CAD build for the part. Positions are in the model's coordinates, mm. A direction names the side the tool comes from. Give positions to 0.01 mm unless a question says otherwise; leave off trailing zeros. Write each loop counter-clockwise with the first axis right and the second up, starting at its lowest first coordinate (ties: lowest second). Pieces come first, ordered by that corner, then holes. Notation, with made-up numbers: (-15.75, -32.5) - (40.25, -32.5) arc R24 ccw to (40.25, -5.5) - close; hole circle Ø6 at (86, 69). An arc over 180 degrees is marked (long way). Answer as a JSON object with one key per item and string values.
Autodesk Inventor part; units mm, degrees
ref_plane "YZ Plane" through (0, 0, 0) normal (1, 0, 0) x (0, 1, 0)
ref_plane "XZ Plane" through (0, 0, 0) normal (0, 1, 0) x (-1, 0, 0)
ref_plane "XY Plane" through (0, 0, 0) normal (0, 0, 1) x (1, 0, 0)
sketch "Sketch1" plane through (0, 0, 0) normal (0, 0, 1) x (1, 0, 0)
  line L0 (-90, -12.5) -> (90, -12.5)
  line L1 (90, -12.5) -> (90, 12.5)
  line L2 (90, 12.5) -> (-90, 12.5)
  line L3 (-90, 12.5) -> (-90, -12.5)
  point P0 (0, 0)
  dimension "d0" = 25
  dimension "d1" = 12.5
  dimension "d2" = 180
  dimension "d3" = 90
extrude "Extrusion1" add sketch "Sketch1" along normal blind 1.6
fillet "Fillet1" radius 3 4 edges at (-90, -12.5, 0.8) (-90, 12.5, 0.8) (90, -12.5, 0.8) (90, 12.5, 0.8)
sketch "Sketch2" plane through (0, 0, 1.6) normal (0, 0, 1) x (1, 0, 0)
  line L0 (-86.5, 9) -> (86.5, 9) construction
  line L1 (86.5, 9) -> (86.5, -9) construction
  line L2 (86.5, -9) -> (-86.5, -9) construction
  line L3 (-86.5, -9) -> (-86.5, 9) construction
  point P0 (0, 0)
  dimension "d7" = 18
  dimension "d8" = 9
  dimension "d9" = 173
  dimension "d10" = 86.5
hole "Hole1" at (-86.5, 9, 1.6) at (-86.5, -9, 1.6) at (86.5, -9, 1.6) at (86.5, 9, 1.6) direction (0, 0, -1) diameter 3.2 end through all
sketch "Sketch4" plane through (0, 0, 1.6) normal (0, 0, 1) x (1, 0, 0)
  line L0 (90, -9.5) -> (90, 9.5)
  line L1 (90, 4) -> (77.5, 4)
  line L2 (77.5, 4) -> (77.5, -4)
  line L3 (77.5, -4) -> (90, -4)
  line L4 (90, -4) -> (90, 4)
  point P0 (0, 0)
  dimension "d20" = 8
  dimension "d21" = 4
  dimension "d22" = 12.5
extrude "Extrusion3" add sketch "Sketch4" along normal blind 6.5
chamfer "Chamfer1" distance 2 angle 45 1 edges at (90, 0, 8.1)
properties part number "SH8_003.1-sunhub8-PCB"
Item 1: Mould opens along Y. For faces 1 (the cylindrical face through (84.914, 9.208, 0.789)), 2 (the cylindrical face through (-89.14, -11.6, 0.81)), 3 (the flat face through (84, 4, 5)) say: +Y half, -Y half, draft (parallel to the pull), parting line (faces both ways), or undercut.
Entries:
{"face 1": "undercut", "face 2": "-Y half", "face 3": "+Y half"}
Item 2: Which spindle directions (+Z, -Z, +X, -X, +Y, -Y) get a long thin tool onto all of the face, cutting with end or side? Do faces 4 (the flat face through (77.5, 0, 5)), 5 (the flat face through (84, -4, 5)), 6 (the flat face through (-1, 0, 0)). Say none if no direction does.
Entries:
{"face 4": "+Z, -X, +Y, -Y", "face 5": "+Z, +X, -X, -Y", "face 6": "-Z, +X, -X, +Y, -Y"}
Item 3: Cut at A-A (y = -2.5). Give the cut face in (x, z), and give its area (3 significant figures).
Entries:
{"outline": "(-90, 0) - (90, 0) - (90, 6.1) - (88, 8.1) - (77.5, 8.1) - (77.5, 1.6) - (-90, 1.6) - close", "area": "367 mm2"}
Item 4: Cut at C-C (x = -61). Give the cut face in (y, z), and give its area (3 significant figures).
Entries:
{"outline": "(-12.5, 0) - (12.5, 0) - (12.5, 1.6) - (-12.5, 1.6) - close", "area": "40.0 mm2"}
Item 5: Flat gauge pins, fed straight in: P1, Ø5, axis at x = -86.5, y = -9, coming from the -Z side; P2, Ø3, axis at y = 0.5, z = 3.5, coming from the -X side; P3, Ø12, axis at x = 25.5, y = -2.5, coming from the +Z side; P4, Ø2, axis at x = 81.5, z = 3.5, coming from the -Y side. Where does each tip first touch, or does it go through?
Entries:
{"P1": "z = 0", "P2": "x = 77.5", "P3": "z = 1.6", "P4": "y = -4"}
Item 6: Cut at B-B (z = 4). Give the cut face in (x, y), and give its area (3 significant figures).
Entries:
{"outline": "(77.5, -4) - (90, -4) - (90, 4) - (77.5, 4) - close", "area": "100 mm2"}
Item 7: Probe line 1 (Y direction, x = 86.5, z = 0.6); line 2 (X direction, y = -9, z = 0.4); line 3 (X direction, y = -8, z = 1.25). List the from-to ranges inside material, lowest first. Write a range as from..to.
Entries:
{"line 1": "-12.5..-10.6, -7.4..7.4, 10.6..12.5", "line 2": "-90..-88.1, -84.9..84.9, 88.1..90", "line 3": "-90..-87.75, -85.25..85.25, 87.75..90"}
